The model under review builds one solid part; all positions refer to its coordinate system, in mm. Coordinates: 2 decimals unless noted, no trailing zeros. Loops run counter-clockwise (first coordinate to the right, second up) from the corner with the lowest first, then second, coordinate; pieces in that order, holes last. Notation, with made-up numbers: M 20,81 L 75,81 A32 ccw 75,114 Z; hole C 50,89 d5. An arc over 180 degrees is marked long. Write item = value, one per line. Start each with the question number.
Q1. Clearance check with a flat-ended pin moving along its axis: pin 1 Ø1.5 at (x, z) = (293, 2) entering from -Y. State where the tip first meets the part, or that it passes through.
Q2. We need section A-A on x = 319.5. Give the boundary of the cut face in (y, z), and give its area (4 significant figures).
Q3. We need section B-B on z = 1.35. Count the separate pieces of the cut face and the enclosed holes in it, and give its area (3 significant figures).
Q4. Wall thickness on probe 1 along Y at (x, z) = (308, 0.9); probe 2 along Y at (x, z) = (327.5, 2.7); probe 3 along Y at (x, z) = (301.5, 0.3): over which ranges is each line inside the solid? List them lowest first.
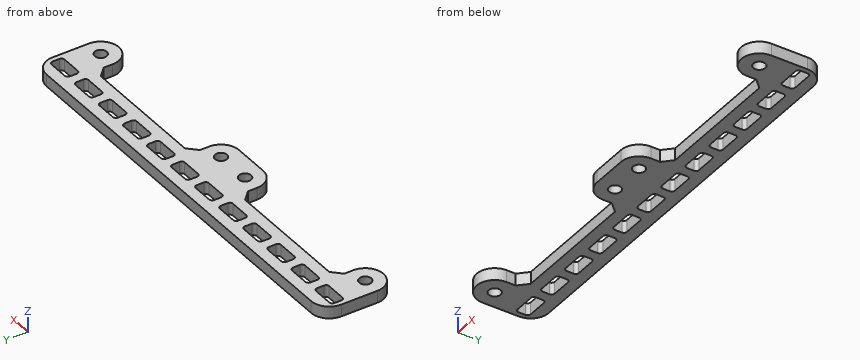
from build123d import *

# Parameters (mm, degrees)
MODEL_R                 = 1.5
SALIENTE_EXTRUIR1_DEPTH = 3


with BuildPart() as part:
    # Model → Saliente-Extruir1 (new body)
    with BuildSketch(Plane.XY):
        with BuildLine():
            Line((256.429131311, 228.742243614), (355.429131311, 228.742243614))
            ThreePointArc((355.429131311, 228.742243614), (358.611111826, 227.424224129), (359.929131311, 224.242243614))
            Line((359.929131311, 224.242243614), (359.929131311, 215.242243614))
            ThreePointArc((359.929131311, 215.242243614), (355.429131311, 210.742243614), (350.929131311, 215.242243614))
            Line((350.929131311, 215.242243614), (350.929131311, 217.492243614))
            Line((350.929131311, 217.492243614), (348.679131311, 219.742243614))
            Line((348.679131311, 219.742243614), (317.179131311, 219.742243614))
            Line((317.179131311, 219.742243614), (314.929131311, 217.492243614))
            Line((314.929131311, 217.492243614), (314.929131311, 215.242243614))
            ThreePointArc((314.929131311, 215.242243614), (313.611111826, 212.060263099), (310.429131311, 210.742243614))
            Line((310.429131311, 210.742243614), (301.429131311, 210.742243614))
            ThreePointArc((301.429131311, 210.742243614), (298.247150795, 212.060263099), (296.929131311, 215.242243614))
            Line((296.929131311, 215.242243614), (296.929131311, 217.492243614))
            Line((296.929131311, 217.492243614), (294.679131311, 219.742243614))
            Line((294.679131311, 219.742243614), (263.179131311, 219.742243614))
            Line((263.179131311, 219.742243614), (260.929131311, 217.492243614))
            Line((260.929131311, 217.492243614), (260.929131311, 215.242243614))
            ThreePointArc((260.929131311, 215.242243614), (256.429131311, 210.742243614), (251.929131311, 215.242243614))
            Line((251.929131311, 215.242243614), (251.929131311, 224.242243614))
            ThreePointArc((251.929131311, 224.242243614), (253.247150795, 227.424224129), (256.429131311, 228.742243614))
        make_face()
        with Locations((301.429131311, 215.242243614)):
            Circle(MODEL_R, mode=Mode.SUBTRACT)
        with Locations((355.429131311, 215.242243614)):
            Circle(MODEL_R, mode=Mode.SUBTRACT)
        with Locations((256.429131311, 215.242243614)):
            Circle(MODEL_R, mode=Mode.SUBTRACT)
        with Locations((310.429131311, 215.242243614)):
            Circle(MODEL_R, mode=Mode.SUBTRACT)
        with BuildLine():
            Line((321.929131311, 222.617243614), (316.929131311, 222.617243614))
            ThreePointArc((316.929131311, 222.617243614), (316.398801225, 222.836913528), (316.179131311, 223.367243614))
            Line((316.179131311, 223.367243614), (316.179131311, 225.117243614))
            ThreePointArc((316.179131311, 225.117243614), (316.398801225, 225.6475737), (316.929131311, 225.867243614))
            Line((316.929131311, 225.867243614), (321.929131311, 225.867243614))
            ThreePointArc((321.929131311, 225.867243614), (322.459461397, 225.6475737), (322.679131311, 225.117243614))
            Line((322.679131311, 225.117243614), (322.679131311, 223.367243614))
            ThreePointArc((322.679131311, 223.367243614), (322.459461397, 222.836913528), (321.929131311, 222.617243614))
        make_face(mode=Mode.SUBTRACT)
        with BuildLine():
            Line((357.929131311, 222.617243614), (352.929131311, 222.617243614))
            ThreePointArc((352.929131311, 222.617243614), (352.398801225, 222.836913528), (352.179131311, 223.367243614))
            Line((352.179131311, 223.367243614), (352.179131311, 225.117243614))
            ThreePointArc((352.179131311, 225.117243614), (352.398801225, 225.6475737), (352.929131311, 225.867243614))
            Line((352.929131311, 225.867243614), (357.929131311, 225.867243614))
            ThreePointArc((357.929131311, 225.867243614), (358.459461397, 225.6475737), (358.679131311, 225.117243614))
            Line((358.679131311, 225.117243614), (358.679131311, 223.367243614))
            ThreePointArc((358.679131311, 223.367243614), (358.459461397, 222.836913528), (357.929131311, 222.617243614))
        make_face(mode=Mode.SUBTRACT)
        with BuildLine():
            Line((348.929131311, 222.617243614), (343.929131311, 222.617243614))
            ThreePointArc((343.929131311, 222.617243614), (343.398801225, 222.836913528), (343.179131311, 223.367243614))
            Line((343.179131311, 223.367243614), (343.179131311, 225.117243614))
            ThreePointArc((343.179131311, 225.117243614), (343.398801225, 225.6475737), (343.929131311, 225.867243614))
            Line((343.929131311, 225.867243614), (348.929131311, 225.867243614))
            ThreePointArc((348.929131311, 225.867243614), (349.459461397, 225.6475737), (349.679131311, 225.117243614))
            Line((349.679131311, 225.117243614), (349.679131311, 223.367243614))
            ThreePointArc((349.679131311, 223.367243614), (349.459461397, 222.836913528), (348.929131311, 222.617243614))
        make_face(mode=Mode.SUBTRACT)
        with BuildLine():
            Line((339.929131311, 222.617243614), (334.929131311, 222.617243614))
            ThreePointArc((334.929131311, 222.617243614), (334.398801225, 222.836913528), (334.179131311, 223.367243614))
            Line((334.179131311, 223.367243614), (334.179131311, 225.117243614))
            ThreePointArc((334.179131311, 225.117243614), (334.398801225, 225.6475737), (334.929131311, 225.867243614))
            Line((334.929131311, 225.867243614), (339.929131311, 225.867243614))
            ThreePointArc((339.929131311, 225.867243614), (340.459461397, 225.6475737), (340.679131311, 225.117243614))
            Line((340.679131311, 225.117243614), (340.679131311, 223.367243614))
            ThreePointArc((340.679131311, 223.367243614), (340.459461397, 222.836913528), (339.929131311, 222.617243614))
        make_face(mode=Mode.SUBTRACT)
        with BuildLine():
            Line((330.929131311, 222.617243614), (325.929131311, 222.617243614))
            ThreePointArc((325.929131311, 222.617243614), (325.398801225, 222.836913528), (325.179131311, 223.367243614))
            Line((325.179131311, 223.367243614), (325.179131311, 225.117243614))
            ThreePointArc((325.179131311, 225.117243614), (325.398801225, 225.6475737), (325.929131311, 225.867243614))
            Line((325.929131311, 225.867243614), (330.929131311, 225.867243614))
            ThreePointArc((330.929131311, 225.867243614), (331.459461397, 225.6475737), (331.679131311, 225.117243614))
            Line((331.679131311, 225.117243614), (331.679131311, 223.367243614))
            ThreePointArc((331.679131311, 223.367243614), (331.459461397, 222.836913528), (330.929131311, 222.617243614))
        make_face(mode=Mode.SUBTRACT)
        with BuildLine():
            Line((289.929131311, 222.617243614), (294.929131311, 222.617243614))
            ThreePointArc((294.929131311, 222.617243614), (295.459461397, 222.836913528), (295.679131311, 223.367243614))
            Line((295.679131311, 223.367243614), (295.679131311, 225.117243614))
            ThreePointArc((295.679131311, 225.117243614), (295.459461397, 225.6475737), (294.929131311, 225.867243614))
            Line((294.929131311, 225.867243614), (289.929131311, 225.867243614))
            ThreePointArc((289.929131311, 225.867243614), (289.398801225, 225.6475737), (289.179131311, 225.117243614))
            Line((289.179131311, 225.117243614), (289.179131311, 223.367243614))
            ThreePointArc((289.179131311, 223.367243614), (289.398801225, 222.836913528), (289.929131311, 222.617243614))
        make_face(mode=Mode.SUBTRACT)
        with BuildLine():
            Line((253.929131311, 222.617243614), (258.929131311, 222.617243614))
            ThreePointArc((258.929131311, 222.617243614), (259.459461397, 222.836913528), (259.679131311, 223.367243614))
            Line((259.679131311, 223.367243614), (259.679131311, 225.117243614))
            ThreePointArc((259.679131311, 225.117243614), (259.459461397, 225.6475737), (258.929131311, 225.867243614))
            Line((258.929131311, 225.867243614), (253.929131311, 225.867243614))
            ThreePointArc((253.929131311, 225.867243614), (253.398801225, 225.6475737), (253.179131311, 225.117243614))
            Line((253.179131311, 225.117243614), (253.179131311, 223.367243614))
            ThreePointArc((253.179131311, 223.367243614), (253.398801225, 222.836913528), (253.929131311, 222.617243614))
        make_face(mode=Mode.SUBTRACT)
        with BuildLine():
            Line((262.929131311, 222.617243614), (267.929131311, 222.617243614))
            ThreePointArc((267.929131311, 222.617243614), (268.459461397, 222.836913528), (268.679131311, 223.367243614))
            Line((268.679131311, 223.367243614), (268.679131311, 225.117243614))
            ThreePointArc((268.679131311, 225.117243614), (268.459461397, 225.6475737), (267.929131311, 225.867243614))
            Line((267.929131311, 225.867243614), (262.929131311, 225.867243614))
            ThreePointArc((262.929131311, 225.867243614), (262.398801225, 225.6475737), (262.179131311, 225.117243614))
            Line((262.179131311, 225.117243614), (262.179131311, 223.367243614))
            ThreePointArc((262.179131311, 223.367243614), (262.398801225, 222.836913528), (262.929131311, 222.617243614))
        make_face(mode=Mode.SUBTRACT)
        with BuildLine():
            Line((271.929131311, 222.617243614), (276.929131311, 222.617243614))
            ThreePointArc((276.929131311, 222.617243614), (277.459461397, 222.836913528), (277.679131311, 223.367243614))
            Line((277.679131311, 223.367243614), (277.679131311, 225.117243614))
            ThreePointArc((277.679131311, 225.117243614), (277.459461397, 225.6475737), (276.929131311, 225.867243614))
            Line((276.929131311, 225.867243614), (271.929131311, 225.867243614))
            ThreePointArc((271.929131311, 225.867243614), (271.398801225, 225.6475737), (271.179131311, 225.117243614))
            Line((271.179131311, 225.117243614), (271.179131311, 223.367243614))
            ThreePointArc((271.179131311, 223.367243614), (271.398801225, 222.836913528), (271.929131311, 222.617243614))
        make_face(mode=Mode.SUBTRACT)
        with BuildLine():
            Line((280.929131311, 222.617243614), (285.929131311, 222.617243614))
            ThreePointArc((285.929131311, 222.617243614), (286.459461397, 222.836913528), (286.679131311, 223.367243614))
            Line((286.679131311, 223.367243614), (286.679131311, 225.117243614))
            ThreePointArc((286.679131311, 225.117243614), (286.459461397, 225.6475737), (285.929131311, 225.867243614))
            Line((285.929131311, 225.867243614), (280.929131311, 225.867243614))
            ThreePointArc((280.929131311, 225.867243614), (280.398801225, 225.6475737), (280.179131311, 225.117243614))
            Line((280.179131311, 225.117243614), (280.179131311, 223.367243614))
            ThreePointArc((280.179131311, 223.367243614), (280.398801225, 222.836913528), (280.929131311, 222.617243614))
        make_face(mode=Mode.SUBTRACT)
        with BuildLine():
            Line((307.929131311, 222.617243614), (312.929131311, 222.617243614))
            ThreePointArc((312.929131311, 222.617243614), (313.459461397, 222.836913528), (313.679131311, 223.367243614))
            Line((313.679131311, 223.367243614), (313.679131311, 225.117243614))
            ThreePointArc((313.679131311, 225.117243614), (313.459461397, 225.6475737), (312.929131311, 225.867243614))
            Line((312.929131311, 225.867243614), (307.929131311, 225.867243614))
            ThreePointArc((307.929131311, 225.867243614), (307.398801225, 225.6475737), (307.179131311, 225.117243614))
            Line((307.179131311, 225.117243614), (307.179131311, 223.367243614))
            ThreePointArc((307.179131311, 223.367243614), (307.398801225, 222.836913528), (307.929131311, 222.617243614))
        make_face(mode=Mode.SUBTRACT)
        with BuildLine():
            Line((298.929131311, 222.617243614), (303.929131311, 222.617243614))
            ThreePointArc((303.929131311, 222.617243614), (304.459461397, 222.836913528), (304.679131311, 223.367243614))
            Line((304.679131311, 223.367243614), (304.679131311, 225.117243614))
            ThreePointArc((304.679131311, 225.117243614), (304.459461397, 225.6475737), (303.929131311, 225.867243614))
            Line((303.929131311, 225.867243614), (298.929131311, 225.867243614))
            ThreePointArc((298.929131311, 225.867243614), (298.398801225, 225.6475737), (298.179131311, 225.117243614))
            Line((298.179131311, 225.117243614), (298.179131311, 223.367243614))
            ThreePointArc((298.179131311, 223.367243614), (298.398801225, 222.836913528), (298.929131311, 222.617243614))
        make_face(mode=Mode.SUBTRACT)
    extrude(amount=SALIENTE_EXTRUIR1_DEPTH)


solid = part.part
Returned:
q1.pin_1 = 219.74
q2.outline = M 219.74,0 L 222.62,0 L 222.62,3 L 219.74,3 Z; M 225.87,0 L 228.74,0 L 228.74,3 L 225.87,3 Z
q2.area = 17.25 mm^2
q3.separate_pieces = 1
q3.enclosed_holes = 16
q3.area = 995 mm^2
q4.probe_1 = 210.74 to 222.62, 225.87 to 228.74
q4.probe_2 = 219.74 to 222.62, 225.87 to 228.74
q4.probe_3 = 210.74 to 213.74, 216.74 to 222.62, 225.87 to 228.74
